Can you work these out from the model? Positions are in its coordinate system, mm. A direction names the side the tool comes from. Coordinates: 2 decimals unless noted, no trailing zeros. Loops run counter-clockwise (first coordinate to the right, second up) from the corner with the lowest first, then second, coordinate; pieces in that order, holes last. Notation, with made-up numbers: M 5,-10 L 58,-10 A12 cw 58,5 Z; hole C 58,-2.5 d10. An arc over 180 degrees is marked long. Answer as a JSON object with one key per item and string values. Group by question number.
Item 1: If I drill on line 1 (X direction, y = -41, z = 11.5); line 2 (Z direction, x = -21, y = 40.5); line 3 (Z direction, x = 321.5, y = -22), over which ranges is the centre line in solid material (lowest first)?
Item 2: I'm going to push a flat-ended pin straight in: pin 1 Ø13 at (y, z) = (-17.5, 34.5) entering from +X. Where does the tip first touch, or does it pass through?
Item 3: Suppose I cut it at A-A (z = 40). Write out the boundary of the cut face in (x, y), then the cut area to 3 significant figures.
Item 4: Suppose I cut it at C-C (x = 301.5). Write out the boundary of the cut face in (y, z), then the cut area to 3 significant figures.
Item 5: Suppose I cut it at B-B (y = 27). Write out the boundary of the cut face in (x, z), then the cut area to 3 significant figures.
Item 6: Which directions (+Z, -Z, +X, -X, +Y, -Y) give clear straight access to the entire face, cutting with the end or side of a thin tool? Please do faces 1 (the flat face through (501.65, -28, 24)), 2 (the cylindrical face through (295.605, -20.846, 26.103)).
```python
from build123d import *

# Parameters (mm, degrees)
F0_W     = 190.5
F0_H     = 98.298
F1_DEPTH = 61.722
F2_R     = 8.89
F3_R     = 7.542044
F4_DEPTH = 406.4


with BuildPart() as f1:
    # F0 (on Top) → F1 (new body)
    with BuildSketch(Plane.XY):
        Rectangle(F0_W, F0_H)
    extrude(amount=F1_DEPTH)

    # F2
    f2_edges = [f1.edges().sort_by_distance(p)[0] for p in [
        (-95.25, 0, 0),
        (0, -49.149, 0),
        (95.25, 0, 0),
        (0, 49.149, 0),
        (95.25, 49.149, 30.861),
        (-95.25, 49.149, 30.861),
        (0, 49.149, 61.722),
        (-95.25, -49.149, 30.861),
        (95.25, -49.149, 30.861),
        (0, -49.149, 61.722),
        (-95.25, 0, 61.722),
        (95.25, 0, 61.722),
    ]]
    fillet(f2_edges, radius=F2_R)

    # F3 (on face) → F4 (join)
    with BuildSketch(Plane.YZ.offset(95.25)):
        with Locations((-28.03967, 23.837732)):
            Circle(F3_R)
    extrude(amount=F4_DEPTH)


solid = f1.part
```
From the geometry:
{
 "1": {"line 1": "-95.22 to 95.22", "line 2": "0 to 61.72", "line 3": "19.32 to 28.35"},
 "2": {"pin 1": "x = 95.25"},
 "3": {"outline": "M -95.25,-40.26 A8.89 ccw -86.36,-49.15 L 86.36,-49.15 A8.89 ccw 95.25,-40.26 L 95.25,40.26 A8.89 ccw 86.36,49.15 L -86.36,49.15 A8.89 ccw -95.25,40.26 Z", "area": "18,700 mm2"},
 "4": {"outline": "C -28.04,23.84 d15.08", "area": "179 mm2"},
 "5": {"outline": "M -95.25,8.89 A8.89 ccw -86.36,0 L 86.36,0 A8.89 ccw 95.25,8.89 L 95.25,52.83 A8.89 ccw 86.36,61.72 L -86.36,61.72 A8.89 ccw -95.25,52.83 Z", "area": "11,700 mm2"},
 "6": {"face 1": "+Z, -Z, +X, +Y, -Y", "face 2": "+X"}
}
